Read the model definition and answer for the solid it produces. Units are mm, in the model's axes. Face numbers are marked on the shaded views. A direction names the side the tool comes from. Give positions to 0.01 mm unless a question says otherwise; leave off trailing zeros. Loops run counter-clockwise (first coordinate to the right, second up) from the corner with the lowest first, then second, coordinate; pieces in that order, holes last. Notation, with made-up numbers: (-39.5, 67) - (-19.5, 67) arc R26 cw to (-19.5, 97) - close; hole circle Ø3 at (24.25, 59). An arc over 180 degrees is marked (long way). Write item = value, one per line.
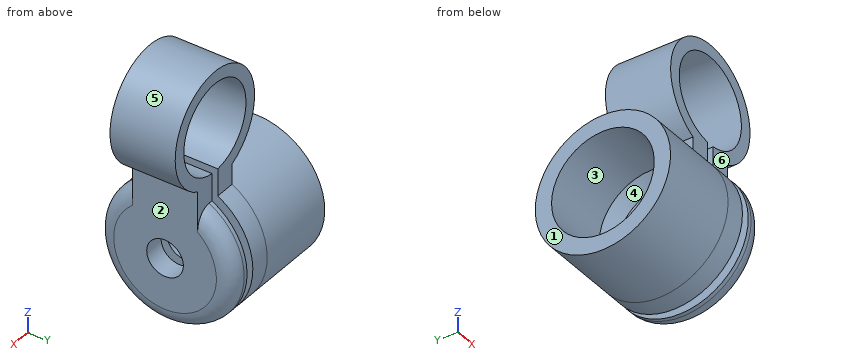
```python
from build123d import *

# Parameters (mm, degrees)
BOSS_EXTRUDE1_DEPTH   = 8
F_8_CLEARANCE_HOLE1_D = 4.4958
SKETCH5_R             = 8.3
SKETCH5_R_2           = 6.3
BOSS_EXTRUDE2_DEPTH   = 10
BOSS_EXTRUDE3_DEPTH   = 2.5
BOSS_EXTRUDE4_START   = 3.5
BOSS_EXTRUDE4_DEPTH   = 2.5
FILLET1_R             = 2
CHAMFER1_SIZE         = 1
CHAMFER1_SIZE2        = 1.732050808


with BuildPart() as part:
    # Sketch1 → Boss-Extrude1 (new body)
    with BuildSketch(Plane(origin=(0, 0, 0), x_dir=(1, 0, 0), z_dir=(0, 1, 0))):
        with BuildLine():
            Line((3, 6.213694553), (3, 20))
            Line((3, 20), (0.5, 20))
            Line((0.5, 20), (0.5, 5.376802024))
            ThreePointArc((0.5, 5.376802024), (0, -5.4), (-0.5, 5.376802024))
            Line((-0.5, 5.376802024), (-0.5, 20))
            Line((-0.5, 20), (-3, 20))
            Line((-3, 20), (-3, 6.213694553))
            ThreePointArc((-3, 6.213694553), (0, -6.9), (3, 6.213694553))
        make_face()
    extrude(amount=BOSS_EXTRUDE1_DEPTH)

    # #8 Clearance Hole1 (through all)
    with Locations(Plane(origin=(3, 0, 0), x_dir=(0, 0, -1), z_dir=(1, 0, 0))):
        with Locations((16, 4)):
            Hole(F_8_CLEARANCE_HOLE1_D / 2)

    # Sketch5 → Boss-Extrude2 (add)
    with BuildSketch(Plane.ZY.offset(3)):
        with Locations(Location((-16, 4, 0), (0, 0, 331.188620291))):
            Circle(SKETCH5_R)
        with Locations(Location((-16, 4, 0), (0, 0, 320.585901644))):
            Circle(SKETCH5_R_2, mode=Mode.SUBTRACT)
    extrude(amount=BOSS_EXTRUDE2_DEPTH)

    # Sketch6 → Boss-Extrude3 (add)
    with BuildSketch(Plane(origin=(-0.5, 0, 0), x_dir=(0, 0, -1), z_dir=(1, 0, 0))):
        with BuildLine():
            Line((20, 0), (8.727448866, 0))
            ThreePointArc((8.727448866, 0), (24.3, 4), (8.727448866, 8))
            Line((8.727448866, 8), (20, 8))
            Line((20, 8), (20, 0))
        make_face()
    extrude(amount=-BOSS_EXTRUDE3_DEPTH)

    # Sketch6<4> → Boss-Extrude4 (add)
    with BuildSketch(Plane(origin=(-0.5, 0, 0), x_dir=(0, 0, -1), z_dir=(1, 0, 0)).offset(BOSS_EXTRUDE4_START)):
        with BuildLine():
            Line((20, 0), (8.727448866, 0))
            ThreePointArc((8.727448866, 0), (24.3, 4), (8.727448866, 8))
            Line((8.727448866, 8), (20, 8))
            Line((20, 8), (20, 0))
        make_face()
    extrude(amount=-BOSS_EXTRUDE4_DEPTH)

    # Fillet1
    fillet1_edges = [part.edges().sort_by_distance(p)[0] for p in [
        (3, 4, -24.3),
    ]]
    fillet(fillet1_edges, radius=FILLET1_R)

    # Chamfer1
    chamfer1_edges = [part.edges().sort_by_distance(p)[0] for p in [
        (-3, 4, -9.7),
    ]]
    chamfer1_side = [part.faces().sort_by_distance(p)[0] for p in [
        (-3, 0.130418557, -15.566381295),
    ]]
    chamfer(chamfer1_edges, length=CHAMFER1_SIZE, length2=CHAMFER1_SIZE2, reference=chamfer1_side[0])


solid = part.part
```
1) A cutting plane is placed at A-A on x = -2.5. Determine the outline of the cut face in (y, z), then the cut area to 3 significant figures.
Output:
outline = (0, -8.73) arc R8.3 ccw (long way) to (8, -8.73) - (8, -4.79) - (0, -4.79) - close; (0, 4.79) - (8, 4.79) - (8, 6.43) - (0, 6.43) - close; hole circle Ø4.5 at (4, -16)
area = 240 mm²
2) Each of these flat-tipped pins is pushed along its axis until it touches: P1, Ø1.5, axis at x = -5.5, z = -20, coming from the -Y side; P2, Ø4, axis at x = -1.5, z = -3.5, coming from the +Y side; P3, Ø1.5, axis at x = -9, z = -1, coming from the -Y side; P4, Ø1, axis at y = 0.5, z = 1.5, coming from the -X side. Where does it stop, or does it pass through?
Output:
P1 = -3.64
P2 = 8
P3 = through
P4 = -6.83
3) A cutting plane is placed at C-C on z = 0. Determine the outline of the cut face in (x, y).
Output:
outline = (-6.9, 0) - (-5.4, 0) - (-5.4, 8) - (-6.9, 8) - close; (5.4, 0) - (6.9, 0) - (6.9, 8) - (5.4, 8) - close
4) A cutting plane is placed at D-D on x = -11.25. Determine the outline of the cut face in (y, z).
Output:
outline = circle Ø16.6 at (4, -16); hole circle Ø12.6 at (4, -16)
5) A tool of negligible diameter and unlimited length cuts with its end or side. For the marked faces 1, 2 and 3, from which of +Z, -Z, +X, -X, +Y, -Y can it reach the whole face along a straight path? Write none if from no direction.
Output:
face_1 = +Z, -Z, -X, +Y, -Y
face_2 = -Z, +X, +Y, -Y
face_3 = -X
6) Find the intervals of material crossed by probe 1 along Z at (x, y) = (-8.5, 4); probe 2 along X at (y, z) = (6, 0); probe 3 along Y at (x, z) = (-2.35, -16), in increasing order.
Output:
probe_1 = -24.3 to -22.3, -9.7 to -7.7
probe_2 = -6.9 to -5.4, 5.4 to 6.9
probe_3 = -4.3 to 1.75, 6.25 to 12.3
7) The mould has two halves that part along Y. Classify the marked faces 4, 5 and 6: pulls with the +Y half, pulls with the -Y half, needs draft (parallel to the pull), parting line crosses it, or undercut.
Output:
face_4 = undercut
face_5 = needs draft
face_6 = pulls with the -Y half
8) A cutting plane is placed at B-B on y = 4. Determine the outline of the cut face in (x, z).
Output:
outline = (-13, -24.3) - (-0.5, -24.3) - (-0.5, -18.25) - (-3, -18.25) - (-3, -21.3) - (-4.73, -22.3) - (-13, -22.3) - close; (-13, -9.7) - (-4.73, -9.7) - (-3, -10.7) - (-3, -13.75) - (-0.5, -13.75) - (-0.5, -5.38) arc R5.4 cw (long way) to (0.5, -5.38) - (0.5, -13.75) - (3, -13.75) - (3, -6.21) arc R6.9 ccw (long way) to (-3, -6.21) - (-3, -7.7) - (-13, -7.7) - close; (0.5, -24.3) - (1, -24.3) arc R2 ccw to (3, -22.3) - (3, -18.25) - (0.5, -18.25) - close
